Build history of the part. All positions in model axes, mm. Coordinates: 2 decimals unless noted, no trailing zeros. Loops run counter-clockwise (first coordinate to the right, second up) from the corner with the lowest first, then second, coordinate; pieces in that order, holes last.
Item 1: Cut at C-C (x = -23). List the corners of the cut face in (y, z).
Item 2: Drill centre lines: line 1 along Y through (x, z) = (11.5, 2.6); line 2 along Y through (x, z) = (7.5, 3.05); line 3 along Y through (x, z) = (-1, 2.75). Where is each one in solid material? Low to high.
Item 3: Cut at D-D (z = 1.6). Count the separate pieces of the cut face and the enclosed holes in it, and give its area (3 significant figures).
Item 4: Cut at B-B (y = 65). List the corners of the cut face in (x, z), and give its area (3 significant figures).
Item 5: Cut at A-A (x = 0). List the corners of the cut face in (y, z), and give its area (3 significant figures).
Item 6: Flat gauge pins, fed straight in: pin 1 (3.5 mm diameter, centred on x = 7.5, y = 55, fed in from -Z); pin 2 (1 mm diameter, centred on y = -14, z = 2, fed in from -X); pin 3 (2 mm diameter, centred on y = 59.5, z = 3, fed in from +X). Where does each tip first touch, or does it go through?
Item 7: Mould opens along Y. For faces 1 (the face through (-0.72, -27.99, 2.46)), 2 (the face through (-20.947, 39.033, 2.465)), 3 (the face through (21.5, 0.07, 2.46)) say: released by +Y, released by -Y, zero draft, split by the parting line, or undercut.
from build123d import *

# Parameters (mm, degrees)
SKETCH1_R           = 1.5
SKETCH1_R_2         = 4
SKETCH1_R_3         = 2
BOSS_EXTRUDE1_DEPTH = 5


with BuildPart() as part:
    # Sketch1 → Boss-Extrude1 (new body)
    with BuildSketch(Plane.XY):
        with BuildLine():
            Line((-15, 70), (-27.062163807, 7.186048295))
            ThreePointArc((-27.062163807, 7.186048295), (0, -28), (27.062163807, 7.186048295))
            Line((27.062163807, 7.186048295), (15, 70))
            Line((15, 70), (-15, 70))
        make_face()
        with Locations((-23, 0)):
            Circle(SKETCH1_R, mode=Mode.SUBTRACT)
        with Locations((-14, 0)):
            Circle(SKETCH1_R, mode=Mode.SUBTRACT)
        with Locations((-11.5, -19.918584287)):
            Circle(SKETCH1_R, mode=Mode.SUBTRACT)
        with Locations((0, -14)):
            Circle(SKETCH1_R, mode=Mode.SUBTRACT)
        with Locations((-11.5, 19.918584287)):
            Circle(SKETCH1_R, mode=Mode.SUBTRACT)
        with BuildLine():
            ThreePointArc((0, 12.5), (-1.5, 14), (0, 15.5))
            ThreePointArc((0, 15.5), (1.5, 14), (0, 12.5))
        make_face(mode=Mode.SUBTRACT)
        with Locations((11.5, -19.918584287)):
            Circle(SKETCH1_R, mode=Mode.SUBTRACT)
        Circle(SKETCH1_R_2, mode=Mode.SUBTRACT)
        with Locations((14, 0)):
            Circle(SKETCH1_R, mode=Mode.SUBTRACT)
        with Locations((23, 0)):
            Circle(SKETCH1_R, mode=Mode.SUBTRACT)
        with Locations((11.5, 19.918584287)):
            Circle(SKETCH1_R, mode=Mode.SUBTRACT)
        with Locations((-7.5, 45)):
            Circle(SKETCH1_R_3, mode=Mode.SUBTRACT)
        with Locations((-7.5, 55)):
            Circle(SKETCH1_R_3, mode=Mode.SUBTRACT)
        with Locations((-7.5, 65)):
            Circle(SKETCH1_R_3, mode=Mode.SUBTRACT)
        with Locations((7.5, 65)):
            Circle(SKETCH1_R_3, mode=Mode.SUBTRACT)
        with Locations((7.5, 55)):
            Circle(SKETCH1_R_3, mode=Mode.SUBTRACT)
        with Locations((7.5, 45)):
            Circle(SKETCH1_R_3, mode=Mode.SUBTRACT)
    extrude(amount=BOSS_EXTRUDE1_DEPTH)


solid = part.part
Filled sheet:
1. outline: (-15.97, 0) - (-1.5, 0) - (-1.5, 5) - (-15.97, 5) - close; (1.5, 0) - (28.34, 0) - (28.34, 5) - (1.5, 5) - close
2. line 1: y = -25.53 to -21.42, -18.42 to 18.42, 21.42 to 70
2. line 2: y = -26.98 to 43, 47 to 53, 57 to 63, 67 to 70
2. line 3: y = -27.98 to -15.12, -12.88 to -3.87, 3.87 to 12.88, 15.12 to 70
3. separate pieces: 1
3. enclosed holes: 17
3. area: 4,080 mm2
4. outline: (-15.96, 0) - (-9.5, 0) - (-9.5, 5) - (-15.96, 5) - close; (-5.5, 0) - (5.5, 0) - (5.5, 5) - (-5.5, 5) - close; (9.5, 0) - (15.96, 0) - (15.96, 5) - (9.5, 5) - close
4. area: 120 mm2
5. outline: (-28, 0) - (-15.5, 0) - (-15.5, 5) - (-28, 5) - close; (-12.5, 0) - (-4, 0) - (-4, 5) - (-12.5, 5) - close; (4, 0) - (12.5, 0) - (12.5, 5) - (4, 5) - close; (15.5, 0) - (70, 0) - (70, 5) - (15.5, 5) - close
5. area: 420 mm2
6. pin 1: passes through
6. pin 2: stops at x = -24.53
6. pin 3: stops at x = 17.21
7. face 1: split by the parting line
7. face 2: released by +Y
7. face 3: undercut
